Autodesk Inventor part; units mm, degrees
ref_plane "YZ Plane" through (0, 0, 0) normal (1, 0, 0) x (0, 1, 0)
ref_plane "XZ Plane" through (0, 0, 0) normal (0, 1, 0) x (-1, 0, 0)
ref_plane "XY Plane" through (0, 0, 0) normal (0, 0, 1) x (1, 0, 0)
sketch "Sketch1" plane through (0, 0, 0) normal (0, 0, 1) x (1, 0, 0)
  circle A0 centre (0, 0) radius 16
  dimension "d0" = 32
extrude "Extrusion1" add sketch "Sketch1" along normal blind 4.5
sketch "Sketch2" plane through (0, 0, 4.5) normal (0, 0, 1) x (1, 0, 0)
  circle A0 centre (0, 0) radius 16
  circle A1 centre (0, 0) radius 8.5
  dimension "d5" = 17
extrude "Extrusion2" add sketch "Sketch2" along normal blind 1 contours A1
sketch "Sketch3" plane through (0, 0, 5.5) normal (0, 0, 1) x (1, 0, 0)
  circle A0 centre (0, 0) radius 8.5
  circle A1 centre (0, 0) radius 7.5
  dimension "d10" = 15
extrude "Extrusion3" cut sketch "Sketch3" against normal through all contours A1
sketch "Sketch4" plane through (0, 0, 4.5) normal (0, 0, 1) x (1, 0, 0)
  circle A0 centre (0, 0) radius 8.5
  circle A1 centre (0, 11.5) radius 1.75
  circle A2 centre (0, 11.5) radius 3
  dimension "d15" = 11.5
  dimension "d16" = 3.5
  dimension "d41" = 6
extrude "Extrusion4" cut sketch "Sketch4" against normal through all contours A1
pattern_circular "Circular Pattern1" count 4 over 360 about axis through (0, 0, 0) along (0, 0, 1) of "Extrusion4"
sketch "Sketch5" plane through (0, 0, 4.5) normal (0, 0, 1) x (1, 0, 0)
  circle A0 centre (0, 11.5) radius 1.75
  circle A1 centre (0, 0) radius 8.5
  arc A2 (0, 8.5) -> (0, 8.5) centre (0, 11.5) ccw
  circle A3 centre (0, 11.5) radius 3
  dimension "d22" = 6
  dimension "d40" = 6
extrude "Extrusion5" cut sketch "Sketch5" against normal blind 3
sketch "Sketch6" plane through (0, 0, 4.5) normal (0, 0, 1) x (1, 0, 0)
  circle A0 centre (-11.5, 0) radius 1.75
  line L0 (-11.5, 3.1754) -> (-8.75, 1.5877)
  line L1 (-8.75, 1.5877) -> (-8.75, -1.5877)
  line L2 (-8.75, -1.5877) -> (-11.5, -3.1754)
  line L3 (-11.5, -3.1754) -> (-14.25, -1.5877)
  line L4 (-14.25, -1.5877) -> (-14.25, 1.5877)
  line L5 (-14.25, 1.5877) -> (-11.5, 3.1754)
  dimension "d28" = 5.5
extrude "Extrusion6" cut sketch "Sketch6" against normal blind 4
pattern_circular "Circular Pattern2" count 2 over 360 about axis through (0, 0, 0) along (0, 0, 1) of "Extrusion6", "Extrusion5"
sketch "Sketch7" plane through (0, 0, 0) normal (0, 0, -1) x (-1, 0, 0)
  circle A0 centre (0, 0) radius 7.5
  circle A1 centre (0, 0) radius 16
  circle A2 centre (0, 0) radius 5
  dimension "d34" = 10
extrude "Extrusion7" add sketch "Sketch7" against normal blind 9 contours A0
properties part number "bearing seat 2"
Geometry: final body of the model. Coordinates: model frame, mm. A direction names the side the tool comes from. Round coordinates to 2 decimals unless told otherwise and drop trailing zeros. Order: outer loops, then holes, each group sorted by start corner. A loop starts at its lowest first (then second) coordinate and runs counter-clockwise, first axis right, second up. Notation, with made-up numbers: M 81.25,-26 L 101.25,-26 A22 ccw 101.25,7 Z; hole C 56.5,26 d10. An arc over 180 degrees is marked long. One line per item, written item: value.
(1) Cut plane C-C (y = 11.5). Return the cut outline in (x, z), and give its area (3 significant figures).
Result sheet:
outline: M -11.12,0 L -1.75,0 L -1.75,1.5 L -3,1.5 L -3,4.5 L -11.12,4.5 Z; M 1.75,0 L 11.12,0 L 11.12,4.5 L 3,4.5 L 3,1.5 L 1.75,1.5 Z
area: 76.9 mm2
(2) Cut plane B-B (x = 4). Return the cut outline in (y, z).
Result sheet:
outline: M -15.49,0 L -3,0 L -3,9 L -6.34,9 L -6.34,5.5 L -7.5,5.5 L -7.5,4.5 L -15.49,4.5 Z; M 3,0 L 15.49,0 L 15.49,4.5 L 7.5,4.5 L 7.5,5.5 L 6.34,5.5 L 6.34,9 L 3,9 Z; hole M -7.5,1.5 L -6.34,1.5 L -6.34,4.5 L -7.5,4.5 Z; hole M 6.34,1.5 L 7.5,1.5 L 7.5,4.5 L 6.34,4.5 Z
(3) Cut plane D-D (z = 7.5). Return the cut outline in (x, y).
Result sheet:
outline: C 0,0 d15; hole C 0,0 d10
(4) Pin query (flat end, axial travel): P1, Ø1.8, axis at x = -0.5, y = 12.5, coming from the +Z side; P2, Ø4, axis at x = 4, z = 5, coming from the +Y side; P3, Ø6, axis at x = -12, y = -0.5, coming from the +Z side. Return the tip coordinate at first contact, or that it passes through.
Result sheet:
P1: z = 1.5
P2: y = 15.87
P3: z = 4.5
(5) Pull-direction query (Y, two-part tool) for faces 4 (the flat face through (-4, 4, 0)), 5 (the cylindrical face through (7.493, 0.33, 7.226)), 6 (the flat face through (-12.8, -1.4, 0.5)); classes: pulls with the +Y half, pulls with the -Y half, needs draft (parallel to the pull), parting line crosses it, or undercut.
Result sheet:
face 4: needs draft
face 5: parting line crosses it
face 6: undercut
(6) Cut plane A-A (z = 2.5). Return the cut outline in (x, y), and give its area (4 significant figures).
Result sheet:
outline: C 0,0 d32; C 0,0 d15; hole M -14.25,-1.59 L -11.5,-3.18 L -8.75,-1.59 L -8.75,1.59 L -11.5,3.18 L -14.25,1.59 Z; hole C 0,0 d17; hole C 0,0 d10; hole C 0,-11.5 d6; hole C 0,11.5 d6; hole M 8.75,-1.59 L 11.5,-3.18 L 14.25,-1.59 L 14.25,1.59 L 11.5,3.18 L 8.75,1.59 Z
area: 566.5 mm2
(7) Line query: probe 1 along X at (y, z) = (-2, 2); probe 2 along Y at (x, z) = (2, 4); probe 3 along Z at (x, y) = (4.5, -8.5). Output: solid intervals per line, ascending. Write a range as [from, to].
Result sheet:
probe 1: [-15.87, -13.54], [-9.46, -8.26], [-7.23, -4.58], [4.58, 7.23], [8.26, 9.46], [13.54, 15.87]
probe 2: [-15.87, -13.74], [-9.26, -8.26], [-7.23, -4.58], [4.58, 7.23], [8.26, 9.26], [13.74, 15.87]
probe 3: [0, 4.5]
(8) Reachability of faces 1 (the cylindrical face through (-0.228, 13.235, 0.76)), 2 (the flat face through (0, -8, 4.5)), 3 (the flat face through (10.106, 2.37, 2.528)) from +Z, -Z, +X, -X, +Y, -Y: full face, straight path, thin tool, end or side. Return the list, or none.
Result sheet:
face 1: +Z, -Z
face 2: none
face 3: +Z
